Work out the finished part from the listing and answer in its coordinate system (mm). A direction names the side the tool comes from. Coordinates: 2 decimals unless noted, no trailing zeros. Order: outer loops, then holes, each group sorted by start corner. A loop starts at its lowest first (then second) coordinate and runs counter-clockwise, first axis right, second up. Notation, with made-up numbers: M -6.5,22.5 L 14.5,22.5 A21 cw 14.5,28.5 Z; hole C 65,-13.5 d1. An arc over 180 degrees is marked long. Use a Markdown table: item, result.
from build123d import *

# Parameters (mm, degrees)
SKETCH1_W           = 69.6
SKETCH1_H           = 69.6
BOSS_EXTRUDE1_DEPTH = 11.6
SKETCH2_W           = 60.7
SKETCH2_H           = 60.6
CUT_EXTRUDE3_DEPTH  = 8.7
SKETCH4_W           = 63.7
SKETCH4_H           = 63.7
CUT_EXTRUDE4_DEPTH  = 1.7
SKETCH5_W           = 8.8
SKETCH5_H           = 2.95
CUT_EXTRUDE5_DEPTH  = 1.7
SKETCH6_W           = 10.090148406
SKETCH6_H           = 10.8025245
SKETCH6_W_2         = 26.487438399
SKETCH6_H_2         = 3.614002098
SKETCH6_W_3         = 9.895864017
CUT_EXTRUDE6_DEPTH  = 7
FILLET1_R           = 3
FILLET2_R           = 1


with BuildPart() as part:
    # Sketch1 → Boss-Extrude1 (new body)
    with BuildSketch(Plane.XY):
        with Locations((34.8, 34.8)):
            Rectangle(SKETCH1_W, SKETCH1_H)
    extrude(amount=BOSS_EXTRUDE1_DEPTH)

    # Sketch2 → Cut-Extrude3 (cut)
    with BuildSketch(Plane.XY.offset(11.6)):
        with Locations((34.8, 34.8)):
            Rectangle(SKETCH2_W, SKETCH2_H)
    extrude(amount=-CUT_EXTRUDE3_DEPTH, mode=Mode.SUBTRACT)

    # Sketch4 → Cut-Extrude4 (cut)
    with BuildSketch(Plane.XY.offset(11.6)):
        with Locations((34.8, 34.8)):
            Rectangle(SKETCH4_W, SKETCH4_H)
    extrude(amount=-CUT_EXTRUDE4_DEPTH, mode=Mode.SUBTRACT)

    # Sketch5 → Cut-Extrude5 (cut)
    with BuildSketch(Plane.XY.offset(11.6)):
        with Locations((11.05, 1.475)):
            Rectangle(SKETCH5_W, SKETCH5_H)
    extrude(amount=-CUT_EXTRUDE5_DEPTH, mode=Mode.SUBTRACT)

    # Sketch6 → Cut-Extrude6 (cut)
    with BuildSketch(Plane.XY.offset(9.9)):
        with Locations((7.995074203, 61.24873775)):
            Rectangle(SKETCH6_W, SKETCH6_H)
        with Locations((40.46662802, 4.757001049)):
            Rectangle(SKETCH6_W_2, SKETCH6_H_2)
        with Locations((61.702067992, 61.24873775)):
            Rectangle(SKETCH6_W_3, SKETCH6_H)
    extrude(amount=-CUT_EXTRUDE6_DEPTH, mode=Mode.SUBTRACT)

    # Fillet1
    fillet1_edges = [part.edges().sort_by_distance(p)[0] for p in [
        (0, 69.6, 5.8),
        (69.6, 69.6, 5.8),
        (69.6, 0, 5.8),
        (0, 0, 5.8),
    ]]
    fillet(fillet1_edges, radius=FILLET1_R)

    # Fillet2
    fillet2_edges = [part.edges().sort_by_distance(p)[0] for p in [
        (11.05, 0, 9.9),
        (15.45, 0, 10.75),
        (6.65, 0, 10.75),
    ]]
    fillet(fillet2_edges, radius=FILLET2_R)


solid = part.part
(1) A cutting plane is placed at B-B (x = 26). Determine the outline of the cut face in (y, z).
Conclusion:
| item | result |
|---|---|
| outline | M 0,0 L 69.6,0 L 69.6,11.6 L 66.65,11.6 L 66.65,9.9 L 65.1,9.9 L 65.1,2.9 L 4.5,2.9 L 4.5,9.9 L 2.95,9.9 L 2.95,11.6 L 0,11.6 Z |
(2) A cutting plane is placed at A-A (z = 7.25). Determine the outline of the cut face in (x, y), then the cut area to 3 significant figures.
Conclusion:
| item | result |
|---|---|
| outline | M 0,3 A3 ccw 3,0 L 66.6,0 A3 ccw 69.6,3 L 69.6,66.6 A3 ccw 66.6,69.6 L 3,69.6 A3 ccw 0,66.6 Z; hole M 2.95,55.85 L 4.45,55.85 L 4.45,4.5 L 27.22,4.5 L 27.22,2.95 L 53.71,2.95 L 53.71,4.5 L 65.15,4.5 L 65.15,55.85 L 66.65,55.85 L 66.65,66.65 L 56.75,66.65 L 56.75,65.1 L 13.04,65.1 L 13.04,66.65 L 2.95,66.65 Z |
| area | 1,060 mm2 |
(3) A cutting plane is placed at C-C (y = 57.5). Determine the outline of the cut face in (x, z).
Conclusion:
| item | result |
|---|---|
| outline | M 0,0 L 69.6,0 L 69.6,11.6 L 66.65,11.6 L 66.65,2.9 L 2.95,2.9 L 2.95,11.6 L 0,11.6 Z |
(4) Straight lines are drawn through the part: L1, parallel to X at y = 42.5, z = 3; L2, parallel to Y at x = 50, z = 9.25; L3, parallel to X at y = 3, z = 3.5. For each, find the intervals that lie inside material, in ascending order.
Conclusion:
| item | result |
|---|---|
| L1 | 0 to 4.45, 65.15 to 69.6 |
| L2 | 0 to 2.95, 65.1 to 69.6 |
| L3 | 0 to 27.22, 53.71 to 69.6 |
(5) A cutting plane is placed at D-D (x = 37.5). Determine the outline of the cut face in (y, z), then the cut area to 3 significant figures.
Conclusion:
| item | result |
|---|---|
| outline | M 0,0 L 69.6,0 L 69.6,11.6 L 66.65,11.6 L 66.65,9.9 L 65.1,9.9 L 65.1,2.9 L 2.95,2.9 L 2.95,11.6 L 0,11.6 Z |
| area | 264 mm2 |
(6) Determine the mould class of faces 1 (the flat face through (0, 34, 6)), 2 (the flat face through (34, 0, 6)), 3 (the flat face through (41, 2.95, 8)) for opening direction Y: pulls with the +Y half, pulls with the -Y half, needs draft (parallel to the pull), parting line crosses it, or undercut.
Conclusion:
| item | result |
|---|---|
| face 1 | needs draft |
| face 2 | pulls with the -Y half |
| face 3 | undercut |
(7) Which of the six approach directions +Z, -Z, +X, -X, +Y, -Y give full straight-line access (tool end or side, diameter ignored) to faces 4 (the flat face through (27.223, 4, 6)), 5 (the cylindrical face through (68.74, 68.7, 5.88))?
Conclusion:
| item | result |
|---|---|
| face 4 | +Z |
| face 5 | +Z, -Z, +X, +Y |
(8) Given P1, Ø1.7, axis at x = 39, y = 65.5, coming from the +Z side; P2, Ø12, axis at x = 19, y = 24, coming from the +Z side; P3, Ø1.4, axis at y = 1.5, z = 10.5, coming from the -X side, each flat-ended and moving along its own axis, determine where each tip first touches the part or whether it passes through.
Conclusion:
| item | result |
|---|---|
| P1 | z = 9.9 |
| P2 | z = 2.9 |
| P3 | x = 0.11 |
